Geometry: final body of the model. Coordinates: model frame, mm. Coordinates: 2 decimals unless noted, no trailing zeros. Write each loop counter-clockwise with the first axis right and the second up, starting at its lowest first coordinate (ties: lowest second). Pieces come first, ordered by that corner, then holes. Notation, with made-up numbers: (56.5, 26) - (84.5, 26) arc R17 cw to (84.5, 47) - close; hole circle Ø9 at (-7, 56). An arc over 180 degrees is marked (long way). Put each result on its own line as item: value.
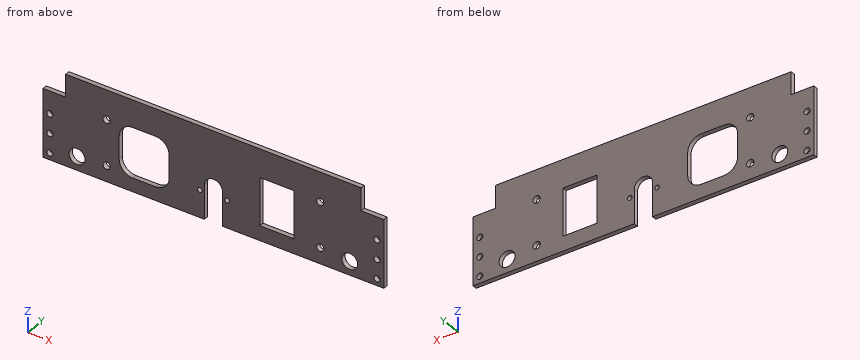
```python
from build123d import *

# Parameters (mm, degrees)
SKETCH_1_R          = 1.35
SKETCH_1_R_2        = 3.5
SKETCH_1_R_3        = 1.6
SKETCH_1_R_4        = 1
SKETCH_1_W          = 22
SKETCH_1_H          = 22
SKETCH_1_W_2        = 15
SKETCH_1_H_2        = 21
EXTRUDE_1_DEPTH     = 2
FILLET_1_R          = 6
SKETCH_2_W          = 16.043978469
SKETCH_2_H          = 25.917195988
CUT_EXTRUDE_1_DEPTH = 79.472925267


with BuildPart() as part:
    # 草图1 → 凸台-拉伸1 (new body)
    with BuildSketch(Plane(origin=(0, 0, 0), x_dir=(1, 0, 0), z_dir=(0, 1, 0))):
        with BuildLine():
            Line((-75, 17), (-4, 17))
            Line((-4, 17), (-4, 2))
            ThreePointArc((-4, 2), (0, -2), (4, 2))
            Line((4, 2), (4, 17))
            Line((4, 17), (75, 17))
            Line((75, 17), (75, -17))
            Line((75, -17), (75, -23))
            Line((75, -23), (-75, -23))
            Line((-75, -23), (-75, -17))
            Line((-75, -17), (-75, 17))
        make_face()
        with Locations(Location((-72, 14, 0), (0, 0, 270))):
            Circle(SKETCH_1_R, mode=Mode.SUBTRACT)
        with Locations(Location((-72, -3, 0), (0, 0, 270))):
            Circle(SKETCH_1_R, mode=Mode.SUBTRACT)
        with Locations(Location((72, -3, 0), (0, 0, 90))):
            Circle(SKETCH_1_R, mode=Mode.SUBTRACT)
        with Locations(Location((72, 14, 0), (0, 0, 90))):
            Circle(SKETCH_1_R, mode=Mode.SUBTRACT)
        with Locations(Location((-60, 11, 0), (0, 0, 270))):
            Circle(SKETCH_1_R_2, mode=Mode.SUBTRACT)
        with Locations(Location((60, 11, 0), (0, 0, 90))):
            Circle(SKETCH_1_R_2, mode=Mode.SUBTRACT)
        with Locations(Location((-47, 10, 0), (0, 0, 270))):
            Circle(SKETCH_1_R_3, mode=Mode.SUBTRACT)
        with Locations(Location((47, 10, 0), (0, 0, 90))):
            Circle(SKETCH_1_R_3, mode=Mode.SUBTRACT)
        with Locations(Location((47, -10, 0), (0, 0, 270))):
            Circle(SKETCH_1_R_3, mode=Mode.SUBTRACT)
        with Locations(Location((-47, -10, 0), (0, 0, 90))):
            Circle(SKETCH_1_R_3, mode=Mode.SUBTRACT)
        with Locations(Location((-6, 5, 0), (0, 0, 270))):
            Circle(SKETCH_1_R_4, mode=Mode.SUBTRACT)
        with Locations(Location((6, 5, 0), (0, 0, 90))):
            Circle(SKETCH_1_R_4, mode=Mode.SUBTRACT)
        with Locations(Location((-72, 5.5, 0), (0, 0, 270))):
            Circle(SKETCH_1_R, mode=Mode.SUBTRACT)
        with Locations(Location((72, 5.5, 0), (0, 0, 90))):
            Circle(SKETCH_1_R, mode=Mode.SUBTRACT)
        with Locations((-30.48, 0)):
            Rectangle(SKETCH_1_W, SKETCH_1_H, mode=Mode.SUBTRACT)
        with Locations((27.94, 0)):
            Rectangle(SKETCH_1_W_2, SKETCH_1_H_2, mode=Mode.SUBTRACT)
    extrude(amount=EXTRUDE_1_DEPTH)

    # 圆角1
    fillet_1_edges = [part.edges().sort_by_distance(p)[0] for p in [
        (-19.48, 1, 11),
        (-19.48, 1, -11),
        (-41.48, 1, -11),
        (-41.48, 1, 11),
    ]]
    fillet(fillet_1_edges, radius=FILLET_1_R)

    # 草图2 → 切除-拉伸1 (cut, through all)
    with BuildSketch(Plane.XZ):
        with Locations((-73.021989235, 25.958597994)):
            Rectangle(SKETCH_2_W, SKETCH_2_H)
        with Locations((73.021989235, 25.958597994)):
            Rectangle(SKETCH_2_W, SKETCH_2_H)
    extrude(amount=-CUT_EXTRUDE_1_DEPTH, mode=Mode.SUBTRACT)


solid = part.part
```
1. Section query A-A (x = 60). Return loops of the section in (y, z), then the cut area to 3 significant figures.
Answer below:
outline: (0, -17) - (2, -17) - (2, -14.5) - (0, -14.5) - close; (0, -7.5) - (2, -7.5) - (2, 23) - (0, 23) - close
area: 66.0 mm²
2. Section query D-D (z = 16.5). Return loops of the section in (x, y), then the cut area to 3 significant figures.
Answer below:
outline: (-65, 0) - (65, 0) - (65, 2) - (-65, 2) - close
area: 260 mm²
3. Ray query, probe 1 along X at (y, z) = (0.65, 3); probe 2 along Z at (x, y) = (-72, 1.05); probe 3 along X at (y, z) = (1, -2.5). Return the intervals inside material, ascending. Write a range as from..to.
Answer below:
probe 1: x = -75..-73.35, -70.65..-41.48, -19.48..20.44, 35.44..70.65, 73.35..75
probe 2: z = -17..-15.35, -12.65..-6.85, -4.15..1.65, 4.35..13
probe 3: x = -75..-41.48, -19.48..-4, 4..20.44, 35.44..75
4. Section query B-B (y = 1.3). Count the separate pieces of the cut face and the enclosed holes in it, then the cut area to 3 significant figures.
Answer below:
separate pieces: 1
enclosed holes: 16
area: 4,740 mm²
5. Section query C-C (x = -38). Return loops of the section in (y, z).
Answer below:
outline: (0, -17) - (2, -17) - (2, -10.45) - (0, -10.45) - close; (0, 10.45) - (2, 10.45) - (2, 23) - (0, 23) - close
